Part model, mm, in its own coordinate system. A direction names the side the tool comes from. Coordinates: 2 decimals unless noted, no trailing zeros. Write each loop counter-clockwise with the first axis right and the second up, starting at its lowest first coordinate (ties: lowest second). Pieces come first, ordered by that corner, then holes. Notation, with made-up numbers: M -1.75,-40 L 36.25,-40 A25 ccw 36.25,-3 Z; hole C 35,85.5 d10. An arc over 180 degrees is marked long. Use a Markdown table: item, result. Add a question column.
Q1. Slice it at C-C on z = 0.7. Count the separate pieces of the cut face and the enclosed holes in it, then the cut area to 3 significant figures.
Q2. Wall check: L1, parallel to Y at x = 43.75, z = 2.5; L2, parallel to X at y = 34.5, z = 1.1; L3, parallel to X at y = 63.5, z = 1.05. Give the ranges that are in metal, low to high. Write a range as from..to.
Q3. Slice it at D-D on y = 12.7. Write the cut outline in (x, z).
Q4. Tool access for faces 1 (the flat face through (32, -51.598, 2)), 2 (the flat face through (44.45, -34, 2)): list every direction of +Z, -Z, +X, -X, +Y, -Y with a clear straight run to the whole face (end or side of a thin tool).
Q5. Slice it at A-A on x = 31.75. Write the cut outline in (y, z) (3 decimals).
Q6. Slice it at B-B on y = -38.1. Write the cut outline in (x, z), then the cut area to 3 significant figures.
Q7. Pin check, flat tip, straight feed: pin 1 Ø2.5 at (x, y) = (19.75, 47.625) entering from -Z. Stop position of the tip, or through.
Autodesk Inventor part; units mm, degrees
ref_plane "YZ Plane" through (0, 0, 0) normal (1, 0, 0) x (0, 1, 0)
ref_plane "XZ Plane" through (0, 0, 0) normal (0, 1, 0) x (-1, 0, 0)
ref_plane "XY Plane" through (0, 0, 0) normal (0, 0, 1) x (1, 0, 0)
sketch "Sketch1" plane through (0, 0, 0) normal (0, 0, 1) x (1, 0, 0)
  line L0 (63.5, 76.2) -> (0, 76.2)
  line L1 (0, 76.2) -> (0, 53.975)
  circle A0 centre (31.75, 47.625) radius 4.05
  line L2 (19.05, -6.35) -> (44.45, -6.35)
  line L3 (63.5, 53.975) -> (63.5, 76.2)
  line L4 (31.75, 76.2) -> (31.75, -6.35)
  circle A1 centre (31.75, 12.7) radius 2.6543
  circle A2 centre (31.75, -12.7) radius 2.6543
  circle A3 centre (31.75, -38.1) radius 2.6604
  line L5 (63.5, 53.975) -> (63.5, -6.35)
  line L6 (63.5, -6.35) -> (0, -6.35)
  line L7 (0, -6.35) -> (0, 53.975)
  line L8 (19.05, -15.3543) -> (19.05, -51.598)
  line L9 (19.05, -51.598) -> (44.45, -51.598)
  line L10 (44.45, -51.598) -> (44.45, -15.3543)
  line L11 (63.5, 53.975) -> (44.45, -15.3543)
  line L12 (0, 53.975) -> (19.05, -15.3543)
  point P0 (0, 0)
  dimension "d0" = 63.5
  dimension "d2" = 8.1
  dimension "d5" = 28.575
  dimension "d50" = 82.55
  dimension "d54" = 5.3086
  dimension "d55" = 63.5
  dimension "d59" = 25.4
  dimension "d60" = 25.4
  dimension "d61" = 25.4
extrude "Extrusion1" add sketch "Sketch1" along normal blind 3.302 contours L3 L11 L6 L2 L4 A1 A0 L0 | L4 A0 A1 L2 L6 L12 L1 L0 | L11 L10 L9 L8 L12 L6 L2
fillet "Fillet11" radius 17.78 1 edges at (63.5, 76.2, 1.651)
fillet "Fillet12" radius 17.78 1 edges at (0, 76.2, 1.651)
sketch "Sketch3" plane through (0, 0, 3.302) normal (0, 0, 1) x (1, 0, 0)
  circle A0 centre (31.75, 47.625) radius 4.05
  circle A1 centre (31.75, 47.625) radius 16
  circle A2 centre (31.75, 47.625) radius 8
  circle A3 centre (31.75, 47.625) radius 12
  line L0 (31.75, 47.625) -> (31.75, 69.8383)
  line L1 (31.75, 47.625) -> (53.9633, 47.625) construction
  point P0 (0, 0)
  point P1 (31.75, 59.625)
  dimension "d28" = 24
  dimension "d26" = 32
  dimension "d27" = 16
  dimension "d36" = 90
hole "Hole1" at (31.75, 59.625, 3.302) direction (0, 0, -1) diameter 4.4958 depth 14.1986 tip angle 118
pattern_circular "Circular Pattern1" count 4 over 360 about axis through (31.75, 47.625, 0) along (0, 0, 1) of "Hole1"
sketch "Sketch4" plane through (0, 0, 3.302) normal (0, 0, 1) x (1, 0, 0)
  circle A0 centre (31.75, 47.625) radius 4.05
  circle A1 centre (31.75, 47.625) radius 12
  circle A2 centre (31.75, 47.625) radius 16
  circle A3 centre (31.75, 47.625) radius 20.955
  line L0 (45.72, 76.2) -> (17.78, 76.2)
  line L1 (31.75, 47.625) -> (51.1677, 67.0427)
  line L2 (31.75, 47.625) -> (59.2107, 47.625) construction
  point P0 (0, 0)
  point P1 (46.5674, 62.4424)
  dimension "d42" = 41.91
  dimension "d40" = 24
  dimension "d41" = 32
  dimension "d58" = 45
hole "Hole2" at (46.5674, 62.4424, 3.302) direction (0, 0, -1) diameter 5.1054 depth 16.256 tip angle 118
pattern_circular "Circular Pattern2" count 4 over 360 about axis through (31.75, 47.625, 0) along (0, 0, 1) of "Hole2"
fillet "Fillet16" radius 6.35 2 edges at (44.45, -15.3543, 1.651) (19.05, -15.3543, 1.651)
equation "\"d54\" = d3"
properties part number "Arm Plate3"
Recorded:
| question | item | result |
|---|---|---|
| 1 | separate pieces | 1 |
| 1 | enclosed holes | 12 |
| 1 | area | 5,010 mm² |
| 2 | L1 | -51.6..45.38, 49.87..76.2 |
| 2 | L2 | 5.35..15.02, 18.84..29.8, 33.7..44.66, 48.48..58.15 |
| 2 | L3 | 0.74..14.61, 19.26..44.24, 48.89..62.76 |
| 3 | outline | M 11.34,0 L 29.1,0 L 29.1,3.3 L 11.34,3.3 Z; M 34.4,0 L 52.16,0 L 52.16,3.3 L 34.4,3.3 Z |
| 4 | face 1 | +Z, -Z, +X, -X, -Y |
| 4 | face 2 | +Z, -Z, +X, -Y |
| 5 | outline | M -51.598,0 L -40.76,0 L -40.76,3.302 L -51.598,3.302 Z; M -35.44,0 L -15.354,0 L -15.354,3.302 L -35.44,3.302 Z; M -10.046,0 L 10.046,0 L 10.046,3.302 L -10.046,3.302 Z; M 15.354,0 L 33.377,0 L 33.377,3.302 L 15.354,3.302 Z; M 37.873,0 L 43.575,0 L 43.575,3.302 L 37.873,3.302 Z; M 51.675,0 L 57.377,0 L 57.377,3.302 L 51.675,3.302 Z; M 61.873,0 L 76.2,0 L 76.2,3.302 L 61.873,3.302 Z |
| 6 | outline | M 19.05,0 L 29.09,0 L 29.09,3.3 L 19.05,3.3 Z; M 34.41,0 L 44.45,0 L 44.45,3.3 L 34.41,3.3 Z |
| 6 | area | 66.3 mm² |
| 7 | pin 1 | through |
